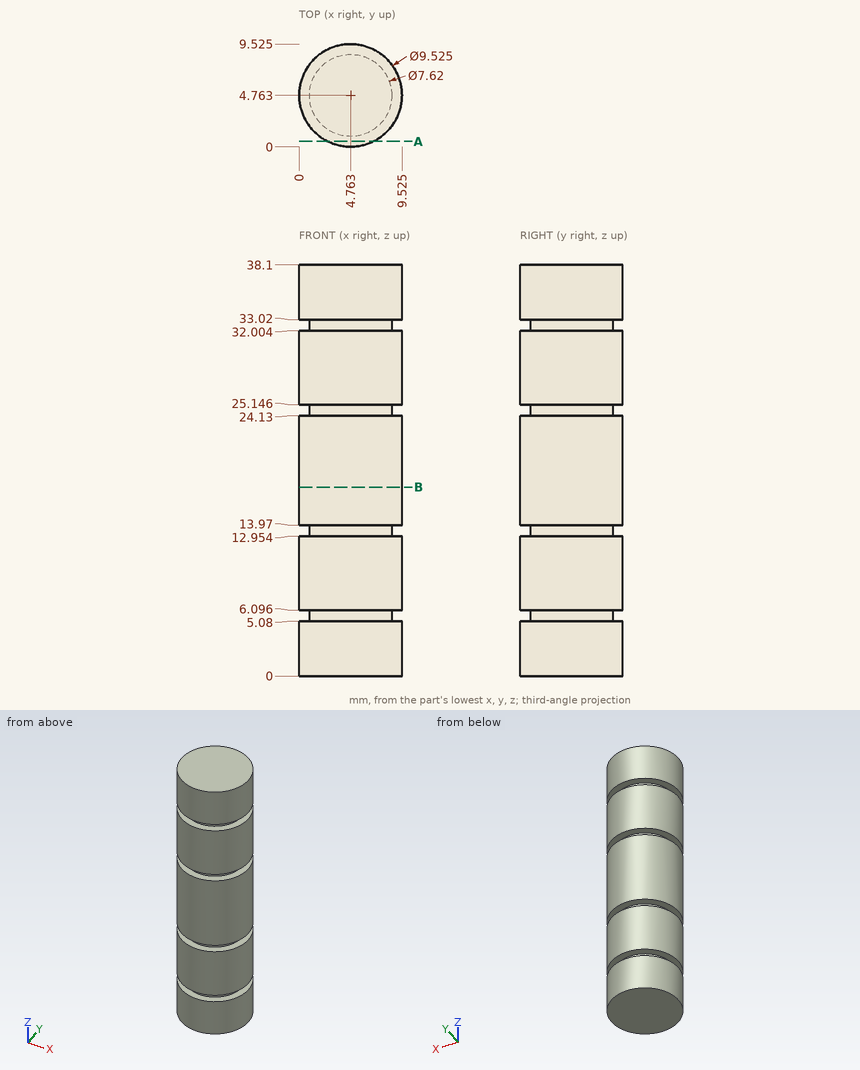
Answer from the drawing. Dimensions are ordinates in mm from the lowest x, y and z of the part. Coordinates: 2 decimals unless noted, no trailing zeros. Loops run counter-clockwise (first coordinate to the right, second up) from the corner with the lowest first, then second, coordinate; pieces in that order, holes last.
1) Consider probe 1 along Z at (x, y) = (9.25, 3.5) (1 decimal); probe 2 along Y at (x, z) = (4.5, 33.5); probe 3 along X at (y, z) = (7, 23) (1 decimal). Determine where each line is inside the solid, lowest interval first.
Results:
probe 1: z = 0 to 5.1, 6.1 to 13, 14 to 24.1, 25.1 to 32, 33 to 38.1
probe 2: y = 0.01 to 9.52
probe 3: x = 0.6 to 9
2) Section B-B (z = 17.5) is taken. Give the vertices of the cut face in (x, y) (1 decimal).
Results:
outline: circle Ø9.5 at (4.8, 4.8)
3) A flat-ended cylindrical pin translates along its axis: pin 1 (4 mm diameter, centred on y = 2.5, z = 28, fed in from +X). Find the tip coordinate at first contact, or state that the pin passes through.
Results:
pin 1: stops at x = 9.52
4) Section A-A (y = 0.5) is taken. Give the vertices of the cut face in (x, z) (1 decimal).
Results:
outline: (2.6, 0) - (6.9, 0) - (6.9, 5.1) - (2.6, 5.1) - close; (2.6, 6.1) - (6.9, 6.1) - (6.9, 13) - (2.6, 13) - close; (2.6, 14) - (6.9, 14) - (6.9, 24.1) - (2.6, 24.1) - close; (2.6, 25.1) - (6.9, 25.1) - (6.9, 32) - (2.6, 32) - close; (2.6, 33) - (6.9, 33) - (6.9, 38.1) - (2.6, 38.1) - close
